For this review, take the finished solid that the model builds, in its own axes (mm). A direction names the side the tool comes from. Give positions to 0.01 mm unless a question says otherwise; leave off trailing zeros. Order: outer loops, then holes, each group sorted by start corner. A loop starts at its lowest first (then second) coordinate and runs counter-clockwise, first axis right, second up. Notation, with made-up numbers: (46, 74) - (63, 74) arc R23 ccw to (63, 108) - close; hole circle Ø2 at (35.5, 74.25). An arc over 180 degrees is marked (long way). One line per item, written item: value.
Autodesk Inventor part; units mm, degrees
ref_plane "YZ Plane" through (0, 0, 0) normal (1, 0, 0) x (0, 1, 0)
ref_plane "XZ Plane" through (0, 0, 0) normal (0, 1, 0) x (-1, 0, 0)
ref_plane "XY Plane" through (0, 0, 0) normal (0, 0, 1) x (1, 0, 0)
sketch "スケッチ1" plane through (0, 0, 0) normal (0, 0, 1) x (1, 0, 0)
  line L0 (-61.5, -20) -> (61.5, -20)
  line L1 (61.5, -20) -> (61.5, 20)
  line L2 (61.5, 20) -> (-61.5, 20)
  line L3 (-61.5, 20) -> (-61.5, -20)
  line L4 (-61.5, -20) -> (61.5, 20) construction
  line L5 (61.5, -20) -> (-61.5, 20) construction
  point P0 (0, 0)
  dimension "d0" = 123
  dimension "d1" = 40
extrude "押し出し1" add sketch "スケッチ1" along normal blind 5
sketch "スケッチ2" plane through (0, 0, 5) normal (0, 0, 1) x (1, 0, 0)
  line L0 (61.5, 20) -> (-61.5, 20)
  line L1 (0, 20) -> (22, 20)
  line L2 (22, 20) -> (22, 5)
  line L3 (22, 5) -> (0, 5)
  line L4 (0, 5) -> (0, 20)
  line L5 (0, 20) -> (-22, 20)
  line L6 (-22, 20) -> (-22, 5)
  line L7 (-22, 5) -> (0, 5)
  line L8 (0, 5) -> (0, 20)
  point P0 (0, 0)
  dimension "d4" = 22
  dimension "d5" = 15
  dimension "d6" = 22
extrude "押し出し2" cut sketch "スケッチ2" against normal blind 5
sketch "スケッチ3" plane through (0, 0, 5) normal (0, 0, 1) x (1, 0, 0)
  line L0 (61.5, 20) -> (22, 20)
  line L1 (-22, 5) -> (-22, 20)
  line L2 (22, 20) -> (22, 5)
  line L3 (-29, 12.5) -> (-55, 12.5) construction
  line L4 (-29, 15.5) -> (-55, 15.5)
  line L5 (-55, 9.5) -> (-29, 9.5)
  arc A0 (-29, 9.5) -> (-29, 15.5) centre (-29, 12.5) ccw
  arc A1 (-55, 15.5) -> (-55, 9.5) centre (-55, 12.5) ccw
  line L6 (55, 12.5) -> (29, 12.5) construction
  line L7 (55, 15.5) -> (29, 15.5)
  line L8 (29, 9.5) -> (55, 9.5)
  arc A2 (55, 9.5) -> (55, 15.5) centre (55, 12.5) ccw
  arc A3 (29, 15.5) -> (29, 9.5) centre (29, 12.5) ccw
  point P0 (0, 0)
  point P1 (42, 12.5)
  point P2 (-42, 12.5)
  dimension "d9" = 7.5
  dimension "d10" = 20
  dimension "d11" = 20
  dimension "d12" = 32
  dimension "d13" = 6
  dimension "d14" = 32
  dimension "d15" = 6
extrude "押し出し3" cut sketch "スケッチ3" against normal blind 5
sketch "スケッチ4" plane through (0, 0, 5) normal (0, 0, 1) x (1, 0, 0)
  line L0 (-61.5, -20) -> (61.5, -20)
  line L1 (61.5, -20) -> (61.5, 20)
  line L2 (-61.5, 20) -> (-61.5, -20)
  point P0 (0, 0)
  point P1 (14.5, -10)
  point P2 (-14.5, -10)
  dimension "d18" = 10
  dimension "d19" = 47
  dimension "d20" = 47
  dimension "d21" = 10
hole "穴1" at (14.5, -10, 5) at (-14.5, -10, 5) direction (0, 0, -1) diameter 5 depth 8.8 tip angle 118
sketch "スケッチ5" plane through (0, 0, 5) normal (0, 0, 1) x (1, 0, 0)
  line L0 (-22, 5) -> (22, 5)
  line L1 (0, 5) -> (-15, 5)
  line L2 (-15, 5) -> (-15, 0)
  line L3 (-15, 0) -> (0, 0)
  line L4 (0, 0) -> (0, 5)
  line L5 (0, 0) -> (15, 0)
  line L6 (15, 0) -> (15, 5)
  line L7 (15, 5) -> (0, 5)
  line L8 (0, 5) -> (0, 0)
  point P0 (0, 0)
  dimension "d29" = 15
  dimension "d30" = 15
extrude "押し出し4" add sketch "スケッチ5" along normal blind 20
sketch "スケッチ6" plane through (-15, 0, 5) normal (0, -1, 0) x (1, 0, 0)
  point P0 (15, -5)
sketch "スケッチ7" plane through (-22, 5, 0) normal (0, 1, 0) x (1, 0, 0)
  line L0 (37, -25) -> (7, -25)
  line L1 (37, -5) -> (37, -25)
  line L2 (7, -5) -> (7, -25)
  point P0 (22, 0)
  point P1 (30, -15)
  point P2 (14, -15)
  dimension "d33" = 10
  dimension "d34" = 10
  dimension "d35" = 7
  dimension "d36" = 7
hole "穴2" at (8, 5, 15) at (-8, 5, 15) direction (0, -1, 0) diameter 5 depth 8.8 tip angle 118
properties part number "20230309gamma"
(1) Take a section at B-B (x = 47.5). Write out the cut boundary in (y, z), then the cut area to 3 significant figures.
Answers below:
outline: (-20, 0) - (9.5, 0) - (9.5, 5) - (-20, 5) - close; (15.5, 0) - (20, 0) - (20, 5) - (15.5, 5) - close
area: 170 mm^2
(2) Take a section at A-A (y = -10). Write out the cut boundary in (x, z), then the cut area to 3 significant figures.
Answers below:
outline: (-61.5, 0) - (-17, 0) - (-17, 5) - (-61.5, 5) - close; (-12, 0) - (12, 0) - (12, 5) - (-12, 5) - close; (17, 0) - (61.5, 0) - (61.5, 5) - (17, 5) - close
area: 565 mm^2
(3) Machinability: for faces 1 (the face through (58, 12.4, 2.5)), 2 (the face through (15, 2, 15)), 3 (the face through (-22, 13, 3)), which of the approach directions +Z, -Z, +X, -X, +Y, -Y give a long, thin tool a straight path to every point of the face, cutting with its end or side? Answer none if there is none.
Answers below:
face 1: +Z, -Z
face 2: +Z, +X, +Y, -Y
face 3: +Z, -Z, +Y
(4) Take a section at C-C (z = 15). Write out the cut boundary in (x, y), then the cut area to 3 significant figures.
Answers below:
outline: (-15, 0) - (-10.5, 0) - (-10.5, 5) - (-15, 5) - close; (-5.5, 0) - (5.5, 0) - (5.5, 5) - (-5.5, 5) - close; (10.5, 0) - (15, 0) - (15, 5) - (10.5, 5) - close
area: 100 mm^2
(5) For P1, Ø8, axis at x = -37, z = 6, coming from the +Y side; P2, Ø6, axis at x = -0.5, y = -14.5, coming from the +Z side; P3, Ø7.5, axis at x = -7.5, z = 18.5, coming from the +Y side; P4, Ø4, axis at x = 8, z = 15, coming from the -Y side, all flat-tipped, find the tip position at first contact; note any pin that passes through.
Answers below:
P1: stops at y = 20
P2: stops at z = 5
P3: stops at y = 5
P4: passes through
(6) Wall thickness on line 1 (X direction, y = 2.3, z = 15); line 2 (Y direction, x = -14.5, z = 2.8); line 3 (X direction, y = -10, z = 1.75): over which ranges is each line inside the solid? List them lowest first. Write a range as from..to.
Answers below:
line 1: x = -15..-10.5, -5.5..5.5, 10.5..15
line 2: y = -20..-12.5, -7.5..5
line 3: x = -61.5..-17, -12..12, 17..61.5
(7) Draft analysis for pull direction Y (two halves, no side actions). For faces 4 (the face through (26, 12.6, 2.5)), 5 (the face through (0, 0, 15)), 6 (the face through (-41, 20, 2)), 7 (the face through (42, 15.5, 3)), state which applies: pulls with the +Y half, pulls with the -Y half, needs draft (parallel to the pull), parting line crosses it, or undercut.
Answers below:
face 4: undercut
face 5: pulls with the -Y half
face 6: pulls with the +Y half
face 7: undercut
(8) Take a section at D-D (x = 8). Write out the cut boundary in (y, z).
Answers below:
outline: (-20, 0) - (5, 0) - (5, 12.5) - (0, 12.5) - (0, 5) - (-20, 5) - close; (0, 17.5) - (5, 17.5) - (5, 25) - (0, 25) - close
